```python
from build123d import *

# Parameters (mm, degrees)
SKETCH_1_W          = 126.5
SKETCH_1_H          = 82.5
SKETCH_1_R          = 2.1
EXTRUDE_1_DEPTH     = 2
CUT_EXTRUDE_1_DEPTH = 0.5
FILLET_1_R          = 1
SKETCH_4_W          = 126.5
SKETCH_4_H          = 82.5
SKETCH_4_R          = 6
EXTRUDE_3_DEPTH     = 3.5


with BuildPart() as part:
    # Эскиз1 → Бобышка-Вытянуть1 (new body)
    with BuildSketch(Plane(origin=(0, 60.645974268, 0), x_dir=(-1, 0, 0), z_dir=(0, -1, 0))):
        with Locations((-64.808980694, -89.523129836)):
            Rectangle(SKETCH_1_W, SKETCH_1_H)
        with Locations(Location((-24.808980694, -59.523129836, 0), (0, 0, 90))):
            Circle(SKETCH_1_R, mode=Mode.SUBTRACT)
        with Locations(Location((-104.808980694, -59.523129836, 0), (0, 0, 90))):
            Circle(SKETCH_1_R, mode=Mode.SUBTRACT)
        with Locations(Location((-24.808980694, -119.523129836, 0), (0, 0, 90))):
            Circle(SKETCH_1_R, mode=Mode.SUBTRACT)
        with Locations(Location((-104.808980694, -119.523129836, 0), (0, 0, 90))):
            Circle(SKETCH_1_R, mode=Mode.SUBTRACT)
    extrude(amount=EXTRUDE_1_DEPTH)

    # Эскиз3 → Вырез-Вытянуть1 (cut)
    with BuildSketch(Plane(origin=(0, 58.645974268, 0), x_dir=(-1, 0, 0), z_dir=(0, -1, 0))):
        Polygon((-59.808980694, -57.523129836), (-32.808980694, -57.523129836), (-32.808980694, -84.523129836), (-12.808980694, -84.523129836), (-12.808980694, -94.523129836), (-32.808980694, -94.523129836), (-32.808980694, -121.523129836), (-59.808980694, -121.523129836), (-59.808980694, -130.773129836), (-69.808980694, -130.773129836), (-69.808980694, -121.523129836), (-96.808980694, -121.523129836), (-96.808980694, -94.523129836), (-116.808980694, -94.523129836), (-116.808980694, -84.523129836), (-96.808980694, -84.523129836), (-96.808980694, -57.523129836), (-69.808980694, -57.523129836), (-69.808980694, -48.273129836), (-59.808980694, -48.273129836), align=None)
    extrude(amount=-CUT_EXTRUDE_1_DEPTH, mode=Mode.SUBTRACT)

    # Скругление1
    fillet_1_edges = [part.edges().sort_by_distance(p)[0] for p in [
        (64.808980694, 59.145974268, 130.773129836),
        (64.808980694, 59.145974268, 48.273129836),
    ]]
    fillet(fillet_1_edges, radius=FILLET_1_R)

    # Эскиз4 → Бобышка-Вытянуть3 (add)
    with BuildSketch(Plane(origin=(0, 60.645974268, 0), x_dir=(-1, 0, 0), z_dir=(0, -1, 0))):
        with Locations((-64.808980694, -89.523129836)):
            Rectangle(SKETCH_4_W, SKETCH_4_H)
        with Locations(Location((-24.808980694, -59.523129836, 0), (0, 0, 90))):
            Circle(SKETCH_4_R, mode=Mode.SUBTRACT)
        with Locations(Location((-104.808980694, -59.523129836, 0), (0, 0, 90))):
            Circle(SKETCH_4_R, mode=Mode.SUBTRACT)
        with Locations(Location((-104.808980694, -119.523129836, 0), (0, 0, 90))):
            Circle(SKETCH_4_R, mode=Mode.SUBTRACT)
        with Locations(Location((-24.808980694, -119.523129836, 0), (0, 0, 90))):
            Circle(SKETCH_4_R, mode=Mode.SUBTRACT)
    extrude(amount=-EXTRUDE_3_DEPTH)


solid = part.part
```
Design review of the part built by this model. Coordinates are the model's own, in mm. A direction names the side the tool comes from. Give positions to 0.01 mm unless a question says otherwise; leave off trailing zeros. Order: outer loops, then holes, each group sorted by start corner. A loop starts at its lowest first (then second) coordinate and runs counter-clockwise, first axis right, second up. Notation, with made-up numbers: M 58.5,49.5 L 80.5,49.5 A22 ccw 80.5,67.5 Z; hole C 78.5,22.25 d9. An arc over 180 degrees is marked long. One line per question, with ' | ' between items. Start each with the question number.
Q1. For pin 1 Ø11 at (x, z) = (24.81, 119.52) entering from +Y, flat-tipped, find the tip position at first contact; note if it passes through.
Q2. For L1, parallel to X at y = 61.4, z = 119; L2, parallel to X at y = 61.15, z = 125; L3, parallel to Z at x = 106, y = 59.6, list the stretches that pass through material, from the lowest coordinate up. Write a range as [from, to].
Q3. We need section D-D (z = 115). Write out the cut boundary in (x, y).
Q4. We need section C-C (y = 62.3). Write out the cut boundary in (x, z).
Q5. Machinability: for faces 5 (the face through (106, 58.646, 80)), 6 (the face through (22, 60.646, 119)), which of the approach directions +Z, -Z, +X, -X, +Y, -Y give a long, thin tool a straight path to every point of the face, cutting with its end or side? Answer none if there is none.
Q6. We need section B-B (x = 87.5). Write out the cut boundary in (y, z), plus the area to 3 significant figures.
Q7. The part is to be moulded in two halves that separate along X. For faces 1 (the face through (128.059, 61, 90)), 2 (the face through (1.559, 61, 90)), 3 (the face through (102, 60.646, 59)), 4 (the face through (102, 60.646, 119)), say which applies: +X half, -X half, draft (parallel to the pull), parting line (faces both ways), or undercut.
Q8. We need section A-A (z = 69). Write out the cut boundary in (x, y).
Returned:
1) pin 1: y = 60.65
2) L1: [1.56, 18.83], [30.79, 98.83], [110.79, 128.06] | L2: [1.56, 22.36], [27.26, 102.36], [107.26, 128.06] | L3: [48.27, 57.79], [61.25, 117.79], [121.25, 130.77]
3) outline: M 1.56,58.65 L 32.81,58.65 L 32.81,59.15 L 96.81,59.15 L 96.81,58.65 L 128.06,58.65 L 128.06,64.15 L 108.75,64.15 L 108.75,60.65 L 100.87,60.65 L 100.87,64.15 L 28.75,64.15 L 28.75,60.65 L 20.87,60.65 L 20.87,64.15 L 1.56,64.15 Z
4) outline: M 1.56,48.27 L 128.06,48.27 L 128.06,130.77 L 1.56,130.77 Z; hole C 24.81,59.52 d12; hole C 24.81,119.52 d12; hole C 104.81,59.52 d12; hole C 104.81,119.52 d12
5) face 5: +Z, -Z, +X, -X, -Y | face 6: +Y
6) outline: M 58.65,48.27 L 64.15,48.27 L 64.15,130.77 L 58.65,130.77 L 58.65,121.52 L 59.15,121.52 L 59.15,57.52 L 58.65,57.52 Z | area: 422 mm2
7) face 1: +X half | face 2: -X half | face 3: undercut | face 4: undercut
8) outline: M 1.56,58.65 L 32.81,58.65 L 32.81,59.15 L 96.81,59.15 L 96.81,58.65 L 128.06,58.65 L 128.06,64.15 L 1.56,64.15 Z
